Source: CAD feature listing. Evaluate the final solid. Frame: model axes, mm. Round coordinates to 2 decimals unless told otherwise and drop trailing zeros. Order: outer loops, then holes, each group sorted by start corner. A loop starts at its lowest first (then second) coordinate and runs counter-clockwise, first axis right, second up. Notation, with made-up numbers: (49, 88.25) - (54, 88.25) arc R15 ccw to (54, 99.25) - close; hole circle Ø1 at (73.5, 8.25). An arc over 180 degrees is marked (long way). Put each result on its own line as item: value. Start each with the question number.
1) Line query: probe 1 along Z at (x, y) = (0, -4) (3 decimals); probe 2 along X at (y, z) = (-1, 1.75); probe 3 along X at (y, z) = (-5.5, -1.5). Output: solid intervals per line, ascending. Write a range as [from, to].
2) Section C-C on y = 0.25. Output: boundary loops of the cut face in (x, z) (3 decimals), then the cut area to 3 significant figures.
3) Section D-D on y = -0.75. Output: boundary loops of the cut face in (x, z) (3 decimals), then the cut area to 3 significant figures.
4) Mould query, pull axis X, two halves, no side actions, for faces 1 (the face through (-1.08, 1.73, 4.88)), 2 (the face through (0, -6, 3)), 3 (the face through (2.456, -2.302, 0.773)). Classes: +X half, -X half, draft (parallel to the pull), parting line (faces both ways), or undercut.
5) Section A-A on x = 0. Output: boundary loops of the cut face in (y, z) (3 decimals), then the cut area to 3 significant figures.
6) Section B-B on z = 0. Output: boundary loops of the cut face in (x, y) (3 decimals).
7) Contact query for flat-ended pins moving along their axis: P1, Ø5, axis at x = -3.5, y = -4.5, coming from the +Z side; P2, Ø1.5, axis at y = 0.5, z = -2.5, coming from the +X side; P3, Ø1, axis at x = -2, z = 1, coming from the +Y side. Output: stop coordinate, or through.
```python
from build123d import *

# Parameters (mm, degrees)
SKETCH1_R           = 5
BOSS_EXTRUDE1_DEPTH = 3.5
SKETCH2_R           = 2.575
CUT_EXTRUDE1_DEPTH  = 3.5
CHAMFER1_SIZE       = 2
SKETCH3_R           = 3.8
BOSS_EXTRUDE2_DEPTH = 6
SKETCH4_R           = 2.575
CUT_EXTRUDE2_DEPTH  = 6


with BuildPart() as part:
    # Sketch1 → Boss-Extrude1 (new body)
    with BuildSketch(Plane(origin=(0, 0, 0), x_dir=(1, 0, 0), z_dir=(0, 1, 0))):
        Circle(SKETCH1_R)
    extrude(amount=BOSS_EXTRUDE1_DEPTH)

    # Sketch2 → Cut-Extrude1 (cut)
    with BuildSketch(Plane(origin=(0, 3.5, 0), x_dir=(1, 0, 0), z_dir=(0, 1, 0))):
        Circle(SKETCH2_R)
    extrude(amount=-CUT_EXTRUDE1_DEPTH, mode=Mode.SUBTRACT)

    # Chamfer1
    chamfer1_edges = [part.edges().sort_by_distance(p)[0] for p in [
        (-2.575, 3.5, 0),
    ]]
    chamfer(chamfer1_edges, length=CHAMFER1_SIZE)

    # Sketch3 → Boss-Extrude2 (add)
    with BuildSketch(Plane.XZ):
        Circle(SKETCH3_R)
    extrude(amount=BOSS_EXTRUDE2_DEPTH)

    # Sketch4 → Cut-Extrude2 (cut)
    with BuildSketch(Plane.XZ.offset(6)):
        Circle(SKETCH4_R)
    extrude(amount=-CUT_EXTRUDE2_DEPTH, mode=Mode.SUBTRACT)


solid = part.part
```
Answer sheet:
1. probe 1: [-3.8, -2.575], [2.575, 3.8]
1. probe 2: [-3.37, -1.89], [1.89, 3.37]
1. probe 3: [-3.49, -2.09], [2.09, 3.49]
2. outline: circle Ø10 at (0, 0); hole circle Ø5.15 at (0, 0)
2. area: 57.7 mm^2
3. outline: circle Ø7.6 at (0, 0); hole circle Ø5.15 at (0, 0)
3. area: 24.5 mm^2
4. face 1: parting line
4. face 2: draft
4. face 3: undercut
5. outline: (-6, -3.8) - (0, -3.8) - (0, -5) - (3.5, -5) - (3.5, -4.575) - (1.5, -2.575) - (-6, -2.575) - close; (-6, 2.575) - (1.5, 2.575) - (3.5, 4.575) - (3.5, 5) - (0, 5) - (0, 3.8) - (-6, 3.8) - close
5. area: 27.7 mm^2
6. outline: (-5, 0) - (-3.8, 0) - (-3.8, -6) - (-2.575, -6) - (-2.575, 1.5) - (-4.575, 3.5) - (-5, 3.5) - close; (2.575, -6) - (3.8, -6) - (3.8, 0) - (5, 0) - (5, 3.5) - (4.575, 3.5) - (2.575, 1.5) - close
7. P1: z = 3.67
7. P2: x = 4.68
7. P3: y = 1.66
